Source: CAD feature listing. Evaluate the final solid. Frame: model axes, mm. A direction names the side the tool comes from. Round coordinates to 2 decimals unless told otherwise and drop trailing zeros. Loops run counter-clockwise (first coordinate to the right, second up) from the corner with the lowest first, then second, coordinate; pieces in that order, holes last.
Item 1: Access query for faces 1 (the flat face through (-84.8, -52.6, 0)), 2 (the flat face through (-95, -25, 0)), 3 (the flat face through (90, -2, 0)). Directions: +Z, -Z, +X, -X, +Y, -Y. A direction counts if a zero-diameter tool reaches every point of the face in a straight line with its end or side. Return the directions, or none.
Item 2: Ray query, L1, parallel to Y at x = 0, z = -1.25; L2, parallel to X at y = 10, z = 0.5; L3, parallel to X at y = -3.5, z = 2.3. Return the intervals inside material, ascending.
Item 3: Section query B-B on x = 0. Return loops of the section in (y, z).
Item 4: Section query D-D on y = -14. Return loops of the section in (x, z), then the cut area to 3 significant figures.
Item 5: Section query A-A on y = 0. Return loops of the section in (x, z).
Item 6: Pull-direction query (Y, two-part tool) for faces 4 (the flat face through (95, -25, 0)), 5 (the flat face through (1, -19, 3)), 6 (the cylindrical face through (-1.172, 8.923, -0.042)); classes: released by +Y, released by -Y, zero draft, split by the parting line, or undercut.
Item 7: Section query C-C on z = -1.8. Return loops of the section in (x, y).
Item 8: First-contact query: P1, Ø1.8, axis at x = -93.5, z = -1.5, coming from the +Y side; P2, Ø1.8, axis at y = -7, z = -1.5, coming from the -X side. Flat tips, straight axial feed; report the tip coordinate or a pass-through.
```python
from build123d import *

# Parameters (mm, degrees)
BOSS_EXTRUDE1_DEPTH      = 3
BOSS_EXTRUDE1_DEPTH_BACK = 3
SKETCH1_R                = 9


with BuildPart() as part:
    # Sketch1 → Boss-Extrude1 (new, two sides: drawn at the far end of the back side and taken through both)
    with BuildSketch(Plane.XY.offset(-BOSS_EXTRUDE1_DEPTH_BACK)):
        Polygon((-90, 20), (90, 20), (90, -25), (100, -25), (100, -45), (70, -60), (-70, -60), (-100, -45), (-100, -25), (-90, -25), align=None)
        Circle(SKETCH1_R, mode=Mode.SUBTRACT)
    extrude(amount=BOSS_EXTRUDE1_DEPTH + BOSS_EXTRUDE1_DEPTH_BACK)


solid = part.part
```
Data:
1. face 1: +Z, -Z, -X, -Y
1. face 2: +Z, -Z, -X, +Y
1. face 3: +Z, -Z, +X, +Y
2. L1: y = -60 to -9, 9 to 20
2. L2: x = -90 to 90
2. L3: x = -90 to -8.29, 8.29 to 90
3. outline: (-60, -3) - (-9, -3) - (-9, 3) - (-60, 3) - close; (9, -3) - (20, -3) - (20, 3) - (9, 3) - close
4. outline: (-90, -3) - (90, -3) - (90, 3) - (-90, 3) - close
4. area: 1,080 mm2
5. outline: (-90, -3) - (-9, -3) - (-9, 3) - (-90, 3) - close; (9, -3) - (90, -3) - (90, 3) - (9, 3) - close
6. face 4: released by +Y
6. face 5: zero draft
6. face 6: undercut
7. outline: (-100, -45) - (-70, -60) - (70, -60) - (100, -45) - (100, -25) - (90, -25) - (90, 20) - (-90, 20) - (-90, -25) - (-100, -25) - close; hole circle Ø18 at (0, 0)
8. P1: stops at y = -25
8. P2: stops at x = -90
